Input: dimensioned drawing with shaded views. Units: mm. Origin: part minimum x, y, z. A direction names the side the tool comes from. Coordinates: 2 decimals unless noted, no trailing zeros. Write each loop counter-clockwise with the first axis right and the second up, starting at its lowest first coordinate (ties: lowest second). Pieces come first, ordered by that corner, then holes. Notation, with made-up numbers: (74, 71.5) -> (117, 71.5) arc R11 ccw to (117, 90.5) -> close; hole circle Ø3 at (-36.75, -29). An arc over 180 degrees is marked (long way). One line per item, written item: value. Start each with the question number.
1. Access query for the marked faces 1 and 2. Directions: +Z, -Z, +X, -X, +Y, -Y. A direction counts if a zero-diameter tool reaches every point of the face in a straight line with its end or side. Return the directions, or none.
2. Section query C-C, the plane z = 14.5. Output: boundary loops of the cut face in (x, y).
3. Section query D-D, the plane x = 60. Output: boundary loops of the cut face in (y, z) (3 decimals).
4. Line query: line 1 (Z direction, x = 24, y = 4.5) (3 decimals); line 2 (X direction, y = 37, z = 19.75); line 3 (X direction, y = 51.5, z = 12.25). Output: solid intervals per line, ascending.
5. Section query A-A, the plane x = 31.75. Output: boundary loops of the cut face in (y, z) (3 decimals), and give its area (3 significant figures).
6. First-contact query: P1, Ø5, axis at x = 40.5, z = 22, coming from the +Y side; P2, Ø4, axis at y = 34, z = 15.5, coming from the -X side; P3, Ø8, axis at y = 36, z = 8.5, coming from the +X side. Flat tips, straight axial feed; report the tip coordinate or a pass-through.
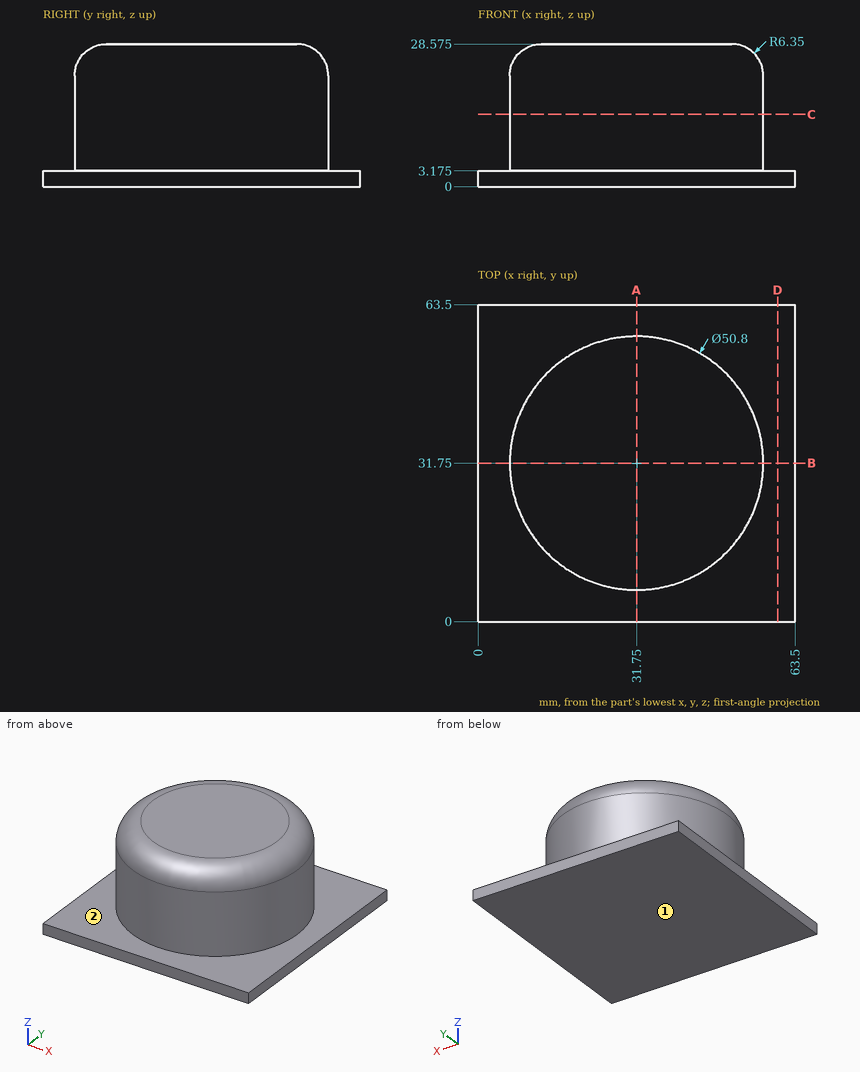
Computed values:
1. face 1: -Z, +X, -X, +Y, -Y
1. face 2: +Z
2. outline: circle Ø50.8 at (31.75, 31.75)
3. outline: (0, 0) -> (63.5, 0) -> (63.5, 3.175) -> (0, 3.175) -> close
4. line 1: z = 0 to 3.175
4. line 2: x = 6.9 to 56.6
4. line 3: x = 15.78 to 47.72
5. outline: (0, 0) -> (63.5, 0) -> (63.5, 3.175) -> (57.15, 3.175) -> (57.15, 22.225) arc R6.35 ccw to (50.8, 28.575) -> (12.7, 28.575) arc R6.35 ccw to (6.35, 22.225) -> (6.35, 3.175) -> (0, 3.175) -> close
5. area: 1,470 mm²
6. P1: stops at y = 56.37
6. P2: stops at x = 6.35
6. P3: stops at x = 57.15
